Could you check a few things on this drawing? It's one solid part, dimensions in mm from its lowest x, y, z. A direction names the side the tool comes from. Give positions to 0.01 mm unless a question says otherwise; leave off trailing zeros. Write each loop counter-clockwise with the first axis right and the second up, starting at its lowest first coordinate (ties: lowest second). Pieces come first, ordered by that corner, then holes.
1. Suppose I cut it at A-A (z = 42.5). Please give me the cut outline in (x, y) (1 decimal).
2. Suppose I cut it at B-B (x = 10.5). Please give me the cut outline in (y, z) (1 decimal), and give its area (3 significant figures).
3. Thinking about a two-plate mould opening in Z: for the marked faces 3, 4 and 5, which applies, pulls with the +Z half, pulls with the -Z half, needs draft (parallel to the pull), parting line crosses it, or undercut?
4. If I drill on probe 1 along Z at (x, y) = (39.5, 10.5) (1 decimal); probe 2 along Y at (x, z) = (14, 16.5); probe 3 along Z at (x, y) = (40, 20.25) (1 decimal), over which ranges is the centre line in solid material (lowest first)?
5. On a 3-axis mill with a long thin cutter (end or side, diameter ignored), from which of +Z, -Z, +X, -X, +Y, -Y can I reach the whole of each face in a straight line? I mean the marked faces 1 and 2. Say none if no direction works.
6. Suppose I cut it at C-C (z = 14). Please give me the cut outline in (x, y) (1 decimal).
7. I'm going to push flat-ended pins straight in: pin 1 (7 mm diameter, centred on x = 25.41, z = 43.89, fed in from -Y); pin 2 (3 mm diameter, centred on y = 6, z = 39, fed in from -X); pin 3 (3 mm diameter, centred on x = 42, z = 23.5, fed in from +Y); pin 4 (3.5 mm diameter, centred on x = 38.47, z = 12.34, fed in from +Y). Where does each tip first touch, or does it pass through?
8. Suppose I cut it at D-D (x = 45). Please give me the cut outline in (y, z).
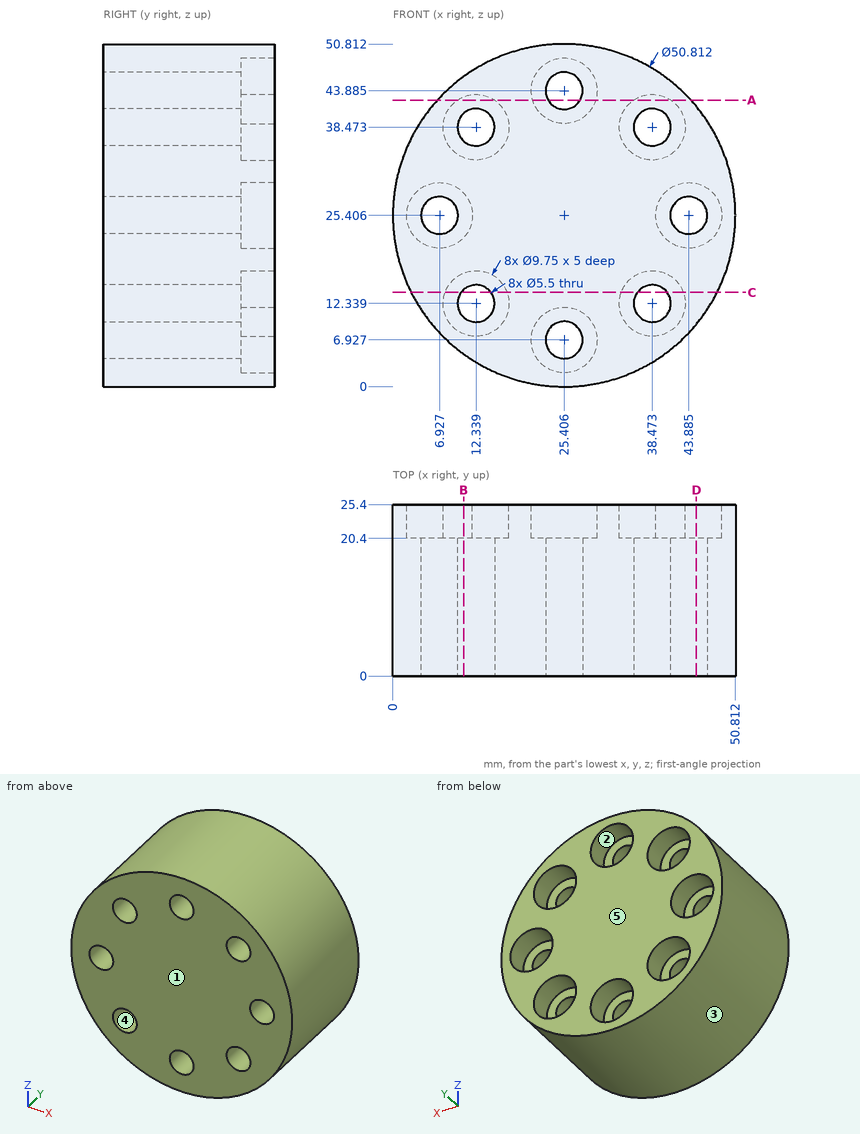
Checks:
1. outline: (6.6, 0) - (23, 0) - (23, 20.4) - (20.7, 20.4) - (20.7, 25.4) - (15.1, 25.4) - (15.1, 20.4) - (9.6, 20.4) - (9.6, 25.4) - (6.6, 25.4) - close; (27.8, 0) - (44.2, 0) - (44.2, 25.4) - (41.2, 25.4) - (41.2, 20.4) - (35.7, 20.4) - (35.7, 25.4) - (30.1, 25.4) - (30.1, 20.4) - (27.8, 20.4) - close
2. outline: (0, 4.8) - (25.4, 4.8) - (25.4, 7.8) - (20.4, 7.8) - (20.4, 10.3) - (0, 10.3) - close; (0, 14.4) - (20.4, 14.4) - (20.4, 16.9) - (25.4, 16.9) - (25.4, 22.1) - (20.4, 22.1) - (20.4, 28.7) - (25.4, 28.7) - (25.4, 34) - (20.4, 34) - (20.4, 36.4) - (0, 36.4) - close; (0, 40.5) - (20.4, 40.5) - (20.4, 43) - (25.4, 43) - (25.4, 46) - (0, 46) - close
2. area: 755 mm2
3. face 3: parting line crosses it
3. face 4: undercut
3. face 5: needs draft
4. probe 1: z = 4.3 to 9.8, 14.9 to 35.9, 41 to 46.5
4. probe 2: y = 0 to 20.4
4. probe 3: z = 4.6 to 10.1, 14.6 to 36.2, 40.8 to 46.2
5. face 1: +Z, -Z, +X, -X, -Y
5. face 2: +Y
6. outline: (2.7, 0) - (10.1, 0) - (10.1, 20.4) - (7.8, 20.4) - (7.8, 25.4) - (2.7, 25.4) - close; (14.5, 0) - (36.3, 0) - (36.3, 20.4) - (33.9, 20.4) - (33.9, 25.4) - (16.9, 25.4) - (16.9, 20.4) - (14.5, 20.4) - close; (40.7, 0) - (48.1, 0) - (48.1, 25.4) - (43.1, 25.4) - (43.1, 20.4) - (40.7, 20.4) - close
7. pin 1: stops at y = 0
7. pin 2: stops at x = 3.06
7. pin 3: stops at y = 20.4
7. pin 4: passes through
8. outline: (0, 9.23) - (25.4, 9.23) - (25.4, 20.66) - (20.4, 20.66) - (20.4, 22.89) - (0, 22.89) - close; (0, 27.92) - (20.4, 27.92) - (20.4, 30.15) - (25.4, 30.15) - (25.4, 41.58) - (0, 41.58) - close
